```python
from build123d import *

# Parameters (mm, degrees)
SKETCH_1_R                    = 9
EXTRUDE_1_DEPTH               = 7.5
EXTRUDE_2_DEPTH               = 8
SKETCH_3_R                    = 11.5
EXTRUDE_3_DEPTH               = 7.5
CHAMFER_2_SIZE                = 0.6
FILLET_1_R                    = 1
HOLE_WIZARD_G1_22_D           = 19
HOLE_WIZARD_G1_22_DEPTH       = 8
HOLE_WIZARD_G1_22_CSINK_D     = 21.005
HOLE_WIZARD_G1_22_CSINK_ANGLE = 90
HOLE_WIZARD_G1_22_TIP         = 5.708175880761822
HOLE_WIZARD_G1_41_D           = 11.8
HOLE_WIZARD_G1_41_DEPTH       = 30.32
HOLE_WIZARD_G1_41_CSINK_D     = 13.207
HOLE_WIZARD_G1_41_CSINK_ANGLE = 90
HOLE_WIZARD_G1_41_TIP         = 3.5450776522626057


with BuildPart() as part:
    # Эскиз1 → Бобышка-Вытянуть1 (new body)
    with BuildSketch(Plane(origin=(0, 0, 0), x_dir=(1, 0, 0), z_dir=(0, 1, 0))):
        with Locations(Location((0, 0, 0), (0, 0, 270))):
            Circle(SKETCH_1_R)
    extrude(amount=EXTRUDE_1_DEPTH)

    # Эскиз2 → Бобышка-Вытянуть2 (add)
    with BuildSketch(Plane(origin=(0, 7.5, 0), x_dir=(1, 0, 0), z_dir=(0, 1, 0))):
        Polygon((-3.47e-15, 13.856406460551018), (-12, 6.92820323027551), (-11.999999999999996, -6.9282032302755105), (1.63e-15, -13.856406460551016), (12, -6.928203230275508), (11.999999999999993, 6.928203230275516), align=None)
    extrude(amount=EXTRUDE_2_DEPTH)

    # Эскиз3 → Бобышка-Вытянуть3 (add)
    with BuildSketch(Plane(origin=(0, 15.5, 0), x_dir=(1, 0, 0), z_dir=(0, 1, 0))):
        with Locations(Location((0, 0, 0), (0, 0, 270))):
            Circle(SKETCH_3_R)
    extrude(amount=EXTRUDE_3_DEPTH)

    # Фаска2
    # the kernel refuses this chamfer: 0.6 mm, written as the material it takes off along each edge
    with BuildSketch(Plane(origin=(13.336285678835246, 7.5, -6.156698333885741), x_dir=(0.01374793830529287, 0.9996219169112968, -0.023812127644089635), z_dir=(-0.8660254037844389, 0, -0.4999999999999997))) as chamfer_2_piece_1:
        Polygon((CHAMFER_2_SIZE * 0.999621916911, -CHAMFER_2_SIZE * 0.0274958766106), (-CHAMFER_2_SIZE * 0.0274958766106, -CHAMFER_2_SIZE * 0.999621916911), (0, 0), align=None)
    extrude(amount=16.942426046110114, mode=Mode.SUBTRACT)
    with BuildSketch(Plane(origin=(1.3362856788352484, 7.5, -14.627911356940793), x_dir=(-0.013747938305293587, 0.9996219169112968, -0.023812127644090856), z_dir=(-0.8660254037844387, 0, 0.5000000000000001))) as chamfer_2_piece_2:
        Polygon((CHAMFER_2_SIZE * 0.999621916911, -CHAMFER_2_SIZE * 0.0274958766106), (-CHAMFER_2_SIZE * 0.0274958766106, -CHAMFER_2_SIZE * 0.999621916911), (0, 0), align=None)
    extrude(amount=16.942426046110114, mode=Mode.SUBTRACT)
    with BuildSketch(Plane(origin=(-12, 7.5, -8.471213023055057), x_dir=(-0.027495876610587344, 0.9996219169112968, 0), z_dir=(2.6e-16, 0, 1))) as chamfer_2_piece_3:
        Polygon((CHAMFER_2_SIZE * 0.999621916911, -CHAMFER_2_SIZE * 0.0274958766106), (-CHAMFER_2_SIZE * 0.0274958766106, -CHAMFER_2_SIZE * 0.999621916911), (0, 0), align=None)
    extrude(amount=16.942426046110118, mode=Mode.SUBTRACT)
    with BuildSketch(Plane(origin=(-13.33628567883525, 7.5, 6.1566983338857355), x_dir=(0.4998109584556482, -0.027495876610585928, -0.8656979742248805), z_dir=(0.8660254037844387, 0, 0.49999999999999983))) as chamfer_2_piece_4:
        Polygon((CHAMFER_2_SIZE * 0.999621916911, CHAMFER_2_SIZE * 0.0274958766106), (-CHAMFER_2_SIZE * 0.0274958766106, CHAMFER_2_SIZE * 0.999621916911), (0, 0), align=None)
    extrude(amount=16.942426046110118, mode=Mode.SUBTRACT)
    with BuildSketch(Plane(origin=(-1.3362856788352513, 7.5, 14.62791135694079), x_dir=(-0.49981095845564827, -0.027495876610585855, -0.8656979742248804), z_dir=(0.8660254037844387, 0, -0.5))) as chamfer_2_piece_5:
        Polygon((CHAMFER_2_SIZE * 0.999621916911, CHAMFER_2_SIZE * 0.0274958766106), (-CHAMFER_2_SIZE * 0.0274958766106, CHAMFER_2_SIZE * 0.999621916911), (0, 0), align=None)
    extrude(amount=16.942426046110114, mode=Mode.SUBTRACT)
    with BuildSketch(Plane(origin=(12, 7.5, 8.471213023055055), x_dir=(-0.9996219169112968, -0.027495876610585904, 0), z_dir=(-5.1e-16, 0, -1))) as chamfer_2_piece_6:
        Polygon((CHAMFER_2_SIZE * 0.999621916911, CHAMFER_2_SIZE * 0.0274958766106), (-CHAMFER_2_SIZE * 0.0274958766106, CHAMFER_2_SIZE * 0.999621916911), (0, 0), align=None)
    extrude(amount=16.94242604611012, mode=Mode.SUBTRACT)
    with BuildSketch(Plane(origin=(13.336285678835246, 15.5, -6.156698333885741), x_dir=(0.01374793830529287, -0.9996219169112968, -0.023812127644089635), z_dir=(-0.8660254037844389, 0, -0.4999999999999997))) as chamfer_2_piece_7_section:
        Polygon((CHAMFER_2_SIZE * 0.999621916911, CHAMFER_2_SIZE * 0.0274958766106), (-CHAMFER_2_SIZE * 0.0274958766106, CHAMFER_2_SIZE * 0.999621916911), (0, 0), align=None)
    chamfer_2_piece_7 = extrude(amount=16.942426046110114, mode=Mode.PRIVATE)
    chamfer_2_piece_7 = chamfer_2_piece_7 - Plane(origin=(0, 15.301333740559118, 0), x_dir=(-1.8e-16, 0, 1), z_dir=(0, -1, 0)) * Cylinder(11.5, 37, mode=Mode.PRIVATE)
    add(chamfer_2_piece_7, mode=Mode.SUBTRACT)
    with BuildSketch(Plane(origin=(1.3362856788352486, 15.5, -14.627911356940793), x_dir=(-0.013747938305293677, -0.9996219169112968, -0.02381212764409101), z_dir=(-0.8660254037844387, 0, 0.5000000000000001))) as chamfer_2_piece_8_section:
        Polygon((CHAMFER_2_SIZE * 0.999621916911, CHAMFER_2_SIZE * 0.0274958766106), (-CHAMFER_2_SIZE * 0.0274958766106, CHAMFER_2_SIZE * 0.999621916911), (0, 0), align=None)
    chamfer_2_piece_8 = extrude(amount=16.942426046110118, mode=Mode.PRIVATE)
    chamfer_2_piece_8 = chamfer_2_piece_8 - Plane(origin=(0, 15.30133374055918, 0), x_dir=(-1.8e-16, 0, 1), z_dir=(0, -1, 0)) * Cylinder(11.5, 37, mode=Mode.PRIVATE)
    add(chamfer_2_piece_8, mode=Mode.SUBTRACT)
    with BuildSketch(Plane(origin=(-12, 15.5, -8.471213023055057), x_dir=(-0.027495876610587344, -0.9996219169112968, 0), z_dir=(2.6e-16, 0, 1))) as chamfer_2_piece_9_section:
        Polygon((CHAMFER_2_SIZE * 0.999621916911, CHAMFER_2_SIZE * 0.0274958766106), (-CHAMFER_2_SIZE * 0.0274958766106, CHAMFER_2_SIZE * 0.999621916911), (0, 0), align=None)
    chamfer_2_piece_9 = extrude(amount=16.942426046110118, mode=Mode.PRIVATE)
    chamfer_2_piece_9 = chamfer_2_piece_9 - Plane(origin=(0, 15.301333740559167, 0), x_dir=(-1.8e-16, 0, 1), z_dir=(0, -1, 0)) * Cylinder(11.5, 37, mode=Mode.PRIVATE)
    add(chamfer_2_piece_9, mode=Mode.SUBTRACT)
    with BuildSketch(Plane(origin=(-13.33628567883525, 15.5, 6.1566983338857355), x_dir=(0.4998109584556481, 0.02749587661058736, -0.8656979742248804), z_dir=(0.8660254037844387, 0, 0.49999999999999983))) as chamfer_2_piece_10_section:
        Polygon((CHAMFER_2_SIZE * 0.999621916911, -CHAMFER_2_SIZE * 0.0274958766106), (-CHAMFER_2_SIZE * 0.0274958766106, -CHAMFER_2_SIZE * 0.999621916911), (0, 0), align=None)
    chamfer_2_piece_10 = extrude(amount=16.942426046110118, mode=Mode.PRIVATE)
    chamfer_2_piece_10 = chamfer_2_piece_10 - Plane(origin=(0, 15.301333740442608, 0), x_dir=(-1.8e-16, 0, 1), z_dir=(0, -1, 0)) * Cylinder(11.5, 37, mode=Mode.PRIVATE)
    add(chamfer_2_piece_10, mode=Mode.SUBTRACT)
    with BuildSketch(Plane(origin=(-1.336285678835251, 15.5, 14.62791135694079), x_dir=(-0.49981095845564827, 0.02749587661058729, -0.8656979742248804), z_dir=(0.8660254037844387, 0, -0.5))) as chamfer_2_piece_11_section:
        Polygon((CHAMFER_2_SIZE * 0.999621916911, -CHAMFER_2_SIZE * 0.0274958766106), (-CHAMFER_2_SIZE * 0.0274958766106, -CHAMFER_2_SIZE * 0.999621916911), (0, 0), align=None)
    chamfer_2_piece_11 = extrude(amount=16.94242604611012, mode=Mode.PRIVATE)
    chamfer_2_piece_11 = chamfer_2_piece_11 - Plane(origin=(0, 15.301333740442338, 0), x_dir=(-1.8e-16, 0, 1), z_dir=(0, -1, 0)) * Cylinder(11.5, 37, mode=Mode.PRIVATE)
    add(chamfer_2_piece_11, mode=Mode.SUBTRACT)
    with BuildSketch(Plane(origin=(12, 15.5, 8.471213023055055), x_dir=(-0.9996219169112968, 0.027495876610587344, 0), z_dir=(-5.1e-16, 0, -1))) as chamfer_2_piece_12_section:
        Polygon((CHAMFER_2_SIZE * 0.999621916911, -CHAMFER_2_SIZE * 0.0274958766106), (-CHAMFER_2_SIZE * 0.0274958766106, -CHAMFER_2_SIZE * 0.999621916911), (0, 0), align=None)
    chamfer_2_piece_12 = extrude(amount=16.94242604611012, mode=Mode.PRIVATE)
    chamfer_2_piece_12 = chamfer_2_piece_12 - Plane(origin=(0, 15.301333740442368, 0), x_dir=(-1.8e-16, 0, 1), z_dir=(0, -1, 0)) * Cylinder(11.5, 37, mode=Mode.PRIVATE)
    add(chamfer_2_piece_12, mode=Mode.SUBTRACT)

    # Скругление1
    fillet_1_edges = [part.edges().sort_by_distance(p)[0] for p in [
        (-3.47e-15, 11.5, -13.856406460551018),
        (11.999999999999993, 11.5, -6.928203230275516),
        (12, 11.5, 6.928203230275508),
        (1.63e-15, 11.5, 13.856406460551016),
        (-11.999999999999996, 11.5, 6.9282032302755105),
        (-12, 11.5, -6.92820323027551),
    ]]
    fillet(fillet_1_edges, radius=FILLET_1_R)

    # Отверстие обработанное метчиком G1/22
    with Locations(Plane(origin=(0, 23, 0), x_dir=(1, 0, 0), z_dir=(0, 1, 0))):
        with Locations((0, 0)):
            CounterSinkHole(HOLE_WIZARD_G1_22_D / 2, HOLE_WIZARD_G1_22_CSINK_D / 2, depth=HOLE_WIZARD_G1_22_DEPTH, counter_sink_angle=HOLE_WIZARD_G1_22_CSINK_ANGLE)
            with Locations((0, 0, -(HOLE_WIZARD_G1_22_DEPTH + HOLE_WIZARD_G1_22_TIP / 2))):  # 118° drill point
                Cone(0, HOLE_WIZARD_G1_22_D / 2, HOLE_WIZARD_G1_22_TIP, mode=Mode.SUBTRACT)

    # Отверстие обработанное метчиком G1/41
    with Locations(Plane(origin=(0, 0, 0), x_dir=(-1, 0, 0), z_dir=(0, -1, 0))):
        with Locations((0, 0)):
            CounterSinkHole(HOLE_WIZARD_G1_41_D / 2, HOLE_WIZARD_G1_41_CSINK_D / 2, depth=HOLE_WIZARD_G1_41_DEPTH, counter_sink_angle=HOLE_WIZARD_G1_41_CSINK_ANGLE)
            with Locations((0, 0, -(HOLE_WIZARD_G1_41_DEPTH + HOLE_WIZARD_G1_41_TIP / 2))):  # 118° drill point
                Cone(0, HOLE_WIZARD_G1_41_D / 2, HOLE_WIZARD_G1_41_TIP, mode=Mode.SUBTRACT)


solid = part.part
```
Work out the finished part from the listing and answer in its coordinate system (mm). A direction names the side the tool comes from. Round coordinates to 2 decimals unless told otherwise and drop trailing zeros. Loops run counter-clockwise (first coordinate to the right, second up) from the corner with the lowest first, then second, coordinate; pieces in that order, holes last. Notation, with made-up numbers: (40, 6.5) -> (47, 6.5) arc R15 ccw to (47, 13.5) -> close; hole circle Ø2 at (16, -32.5). An arc over 180 degrees is marked (long way). Write each question's results on one line, items separated by ' | '. Start each with the question number.
1. Find the intervals of material crossed by probe 1 along Z at (x, y) = (0, 20.5); probe 2 along Y at (x, z) = (8, 7.5); probe 3 along Y at (x, z) = (10.5, -7), in increasing order. Write a range as from..to.
2. Section C-C (z = 11) is taken. Determine the outline of the cut face in (x, y), plus the area to 3 significant figures.
3. Given pin 1 Ø10.5 at (x, z) = (0, 0) entering from +Y; pin 2 Ø1 at (y, z) = (17.5, -10) entering from +X; pin 3 Ø2 at (y, z) = (13.5, -8) entering from -X; pin 4 Ø3 at (x, y) = (3.5, 20) entering from -Z, each flat-ended and moving along its own axis, determine where each tip first touches the part or whether it passes through.
4. Section B-B (y = 20.5) is taken. Determine the outline of the cut face in (x, z), plus the area to 3 significant figures.
5. For a pull along Z with two mould halves and no side action, classify faces 1 (the face through (0, 11.5, -13.7)), 2 (the face through (-4.38, 18.45, 8.43)), 3 (the face through (5.765, 7.796, 10.177)) as +Z half, -Z half, draft (parallel to the pull), parting line (faces both ways), or undercut.
6. Section A-A (z = 0) is taken. Determine the outline of the cut face in (x, y), plus the area to 3 significant figures.
7. A tool of negligible diameter and unlimited length cuts with its end or side. For faces 4 (the face through (-10, 15.5, -6)), 5 (the face through (-7, 7.5, -6)), 6 (the face through (-10.2, 23, 3.4)), from which of +Z, -Z, +X, -X, +Y, -Y can it reach the whole face along a straight path? Write none if from no direction.
Evaluation:
1) probe 1: z = -11.5..-9.5, 9.5..11.5 | probe 2: y = 7.5..23 | probe 3: y = 7.5..15.5
2) outline: (-4.95, 8.1) -> (-3.75, 7.5) -> (3.75, 7.5) -> (4.95, 8.1) -> (4.95, 14.9) -> (3.75, 15.5) -> (3.35, 15.5) -> (3.35, 23) -> (-3.35, 23) -> (-3.35, 15.5) -> (-3.75, 15.5) -> (-4.95, 14.9) -> close | area: 128 mm2
3) pin 1: passes through | pin 2: stops at x = 6.48 | pin 3: stops at x = -11.76 | pin 4: stops at z = -11.32
4) outline: circle Ø23 at (0, 0); hole circle Ø19 at (0, 0) | area: 132 mm2
5) face 1: -Z half | face 2: undercut | face 3: +Z half
6) outline: (-12, 8.1) -> (-11.4, 7.5) -> (-9, 7.5) -> (-9, 0) -> (-6.6, 0) -> (-5.9, 0.7) -> (-5.9, 12.84) -> (-9.5, 15) -> (-9.5, 22) -> (-10.5, 23) -> (-11.5, 23) -> (-11.5, 15.4) -> (-12, 14.9) -> close; (5.9, 0.7) -> (6.6, 0) -> (9, 0) -> (9, 7.5) -> (11.4, 7.5) -> (12, 8.1) -> (12, 14.9) -> (11.5, 15.4) -> (11.5, 23) -> (10.5, 23) -> (9.5, 22) -> (9.5, 15) -> (5.9, 12.84) -> close | area: 161 mm2
7) face 4: -Z, -X, +Y | face 5: -Y | face 6: +Z, -Z, +X, -X, +Y
